from build123d import *

# Parameters (mm, degrees)
SKETCH1_W           = 13
SKETCH1_H           = 23
BOSS_EXTRUDE1_DEPTH = 4
BOSS_EXTRUDE2_DEPTH = 5
CUT_EXTRUDE1_REACH  = 49.476
CUT_EXTRUDE2_REACH  = 35.392
SKETCH4_W           = 5
SKETCH4_H           = 5
SKETCH4_W_2         = 2
SKETCH4_H_2         = 2.5
SKETCH5_W           = 2
SKETCH5_H           = 4
BOSS_EXTRUDE3_DEPTH = 4
CUT_EXTRUDE3_REACH  = 40.859
SKETCH6_R           = 1


with BuildPart() as part:
    # Sketch1 → Boss-Extrude1 (new body)
    with BuildSketch(Plane(origin=(0, 0, 0), x_dir=(1, 0, 0), z_dir=(0, 1, 0))):
        with BuildLine():
            Line((-8, -19), (8, -19))
            ThreePointArc((8, -19), (27, 0), (8, 19))
            Line((8, 19), (-8, 19))
            Line((-8, 19), (-8, -19))
        make_face()
        with BuildLine():
            Line((8, 17), (8, -17))
            ThreePointArc((8, -17), (25, 0), (8, 17))
        make_face(mode=Mode.SUBTRACT)
        with Locations((0, -5)):
            Rectangle(SKETCH1_W, SKETCH1_H, mode=Mode.SUBTRACT)
    extrude(amount=BOSS_EXTRUDE1_DEPTH)

    # Sketch2 → Boss-Extrude2 (add)
    with BuildSketch(Plane(origin=(0, 4, 0), x_dir=(1, 0, 0), z_dir=(0, 1, 0))):
        with BuildLine():
            Line((8, 19), (8, 17))
            ThreePointArc((8, 17), (25, 0), (8, -17))
            Line((8, -17), (8, -19))
            ThreePointArc((8, -19), (27, 0), (8, 19))
        make_face()
    extrude(amount=BOSS_EXTRUDE2_DEPTH)

    # Cut-Extrude1: up to this face of the body (flat: up to its plane)
    cut_extrude1_end = Plane(part.part.faces().sort_by_distance((0, 2, -19))[0])
    # Sketch3 → Cut-Extrude1 (cut, up to the picked face)
    with BuildSketch(Plane.XY.offset(19), mode=Mode.PRIVATE) as cut_extrude1_sk1:
        Polygon((8, 4), (8, 9), (16.660254038, 9), align=None)
    cut_extrude1_tool1 = split(extrude(cut_extrude1_sk1.sketch, amount=-CUT_EXTRUDE1_REACH, mode=Mode.PRIVATE), bisect_by=cut_extrude1_end, keep=Keep.BOTH, mode=Mode.PRIVATE)
    # Sketch3 → Cut-Extrude1 (cut, up to the picked face)
    with BuildSketch(Plane.XY.offset(19), mode=Mode.PRIVATE) as cut_extrude1_sk2:
        Polygon((27, 7), (14.875644347, 0), (27, 0), align=None)
    cut_extrude1_tool2 = split(extrude(cut_extrude1_sk2.sketch, amount=-CUT_EXTRUDE1_REACH, mode=Mode.PRIVATE), bisect_by=cut_extrude1_end, keep=Keep.BOTH, mode=Mode.PRIVATE)
    add(cut_extrude1_tool1.solids().sort_by(Axis((10.886751, 7.333333, 19), (0, 0, -1)))[0], mode=Mode.SUBTRACT)
    add(cut_extrude1_tool2.solids().sort_by(Axis((22.958548, 2.333333, 19), (0, 0, -1)))[0], mode=Mode.SUBTRACT)

    # Sketch4 → Cut-Extrude2 (cut, up to next)
    with BuildSketch(Plane(origin=(0, 4, 0), x_dir=(1, 0, 0), z_dir=(0, 1, 0)), mode=Mode.PRIVATE) as cut_extrude2_sk1:
        with Locations((0, 9)):
            Rectangle(SKETCH4_W, SKETCH4_H)
    cut_extrude2_tool1 = extrude(cut_extrude2_sk1.sketch, amount=-CUT_EXTRUDE2_REACH, mode=Mode.PRIVATE) & part.part
    # Sketch4 → Cut-Extrude2 (cut, up to next)
    with BuildSketch(Plane(origin=(0, 4, 0), x_dir=(1, 0, 0), z_dir=(0, 1, 0)), mode=Mode.PRIVATE) as cut_extrude2_sk2:
        with Locations((0, -17.75)):
            Rectangle(SKETCH4_W_2, SKETCH4_H_2)
    cut_extrude2_tool2 = extrude(cut_extrude2_sk2.sketch, amount=-CUT_EXTRUDE2_REACH, mode=Mode.PRIVATE) & part.part
    add(cut_extrude2_tool1.solids().sort_by_distance((0, 4, -9))[0], mode=Mode.SUBTRACT)
    add(cut_extrude2_tool2.solids().sort_by_distance((0, 4, 17.75))[0], mode=Mode.SUBTRACT)

    # Sketch5 → Boss-Extrude3 (add)
    with BuildSketch(Plane.XZ):
        with Locations((-2, 21)):
            Rectangle(SKETCH5_W, SKETCH5_H)
    boss_extrude3 = extrude(amount=-BOSS_EXTRUDE3_DEPTH)

    # Sketch6 → Cut-Extrude3 (cut, up to next)
    with BuildSketch(Plane.ZY.offset(3), mode=Mode.PRIVATE) as cut_extrude3_sk1:
        with Locations((21, 2)):
            Circle(SKETCH6_R)
    cut_extrude3_tool1 = extrude(cut_extrude3_sk1.sketch, amount=-CUT_EXTRUDE3_REACH, mode=Mode.PRIVATE) & part.part
    cut_extrude3 = cut_extrude3_tool1.solids().sort_by_distance((-3, 2, 21))[0]
    add(cut_extrude3, mode=Mode.SUBTRACT)

    # Mirror1: Boss-Extrude3, Cut-Extrude3 across plane
    add(boss_extrude3.mirror(Plane(origin=(0, 0, 0), x_dir=(0, 0, 1), z_dir=(1, 0, 0))))
    add(cut_extrude3.mirror(Plane(origin=(0, 0, 0), x_dir=(0, 0, 1), z_dir=(1, 0, 0))), mode=Mode.SUBTRACT)


solid = part.part
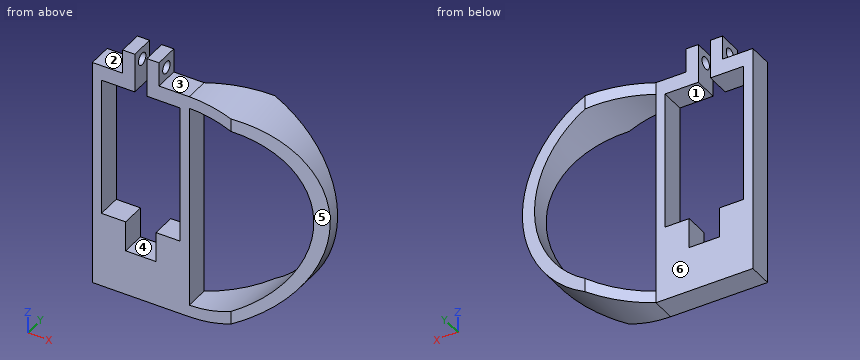
Source: CAD feature listing. Evaluate the final solid. Frame: model axes, mm. Face numbers are marked on the shaded views. A direction names the side the tool comes from. Round coordinates to 2 decimals unless told otherwise and drop trailing zeros. Write each loop counter-clockwise with the first axis right and the second up, starting at its lowest first coordinate (ties: lowest second). Pieces come first, ordered by that corner, then holes. Notation, with made-up numbers: (43.5, 3.25) - (85.5, 3.25) arc R20 cw to (85.5, 41.25) - close; hole circle Ø3 at (38, -3). An arc over 180 degrees is marked (long way). Use CSV: the item, a comma, the result in double quotes. Start each with the question number.
(1) First-contact query: pin 1 Ø3 at (y, z) = (1, -9) entering from +X; pin 2 Ø4 at (x, y) = (8, 6.5) entering from +Z; pin 3 Ø1 at (y, z) = (6, 11.5) entering from +X; pin 4 Ø3 at (y, z) = (6, -11.5) entering from -X. Flat tips, straight axial feed; report the tip coordinate or a pass-through.
(2) Set-up query: the marked faces 1, 2 and 3. Return all of +Z, -Z, +X, -X, +Y, -Y with unobstructed straight access to the full face (end or side cutting, diameter ignored); none if empty.
(3) Material intervals for probe 1 along Y at (x, z) = (1.45, 21); probe 2 along X at (y, z) = (1.5, 6); probe 3 along Z at (x, y) = (5.5, 2.5), sorted ascending. Write a range as [from, to].
(4) Mould query, pull axis X, two halves, no side actions, for the marked faces 4, 5 and 6. Classes: pulls with the +X half, pulls with the -X half, needs draft (parallel to the pull), parting line crosses it, or undercut.
(5) Cut plane D-D, the plane y = 5.5. Return loops of the section in (x, z).
(6) Cut plane A-A, the plane z = 21. Return loops of the section in (x, y).
(7) Cut plane B-B, the plane x = 11.5. Return loops of the section in (y, z), and give its area (3 significant figures).
(8) Cut plane C-C, the plane z = -6. Return loops of the section in (x, y), and give its area (3 significant figures).
Geometry says:
1,pin 1,"x = 8"
1,pin 2,"through"
1,pin 3,"x = 23.49"
1,pin 4,"x = 18.95"
2,face 1,"+Y, -Y"
2,face 2,"+Z, -X, +Y, -Y"
2,face 3,"+Z, +X, +Y, -Y"
3,probe 1,"[0, 1], [3, 4]"
3,probe 2,"[-8, -6.5], [6.5, 8]"
3,probe 3,"[-19, -6.5], [16.5, 19]"
4,face 4,"undercut"
4,face 5,"pulls with the +X half"
4,face 6,"needs draft"
5,outline,"(10.6, -18.82) arc R19 ccw to (24.4, -9.59) - (24.4, -4.47) arc R17 cw to (10.6, -16.8) - close; (10.6, 16.8) arc R17 cw to (24.4, 4.47) - (24.4, 9.59) arc R19 ccw to (10.6, 18.82) - close"
6,outline,"(-3, 0) - (-1, 0) - (-1, 1) - (-3, 1) - close; (-3, 3) - (-1, 3) - (-1, 4) - (-3, 4) - close; (1, 0) - (3, 0) - (3, 1) - (1, 1) - close; (1, 3) - (3, 3) - (3, 4) - (1, 4) - close"
7,outline,"(0, -18.67) - (6.02, -18.67) - (6.02, -16.64) - (0, -16.64) - close; (0, 16.64) - (6.02, 16.64) - (6.02, 18.67) - (0, 18.67) - close"
7,area,"24.6 mm²"
8,outline,"(-8, 0) - (-6.5, 0) - (-6.5, 4) - (-8, 4) - close; (6.5, 0) - (8, 0) - (8, 4) - (6.5, 4) - close; (23.91, 5.21) - (26.03, 6.44) - (26.03, 9) - (23.91, 9) - close"
8,area,"18.7 mm²"
